The drawing under review shows one solid part. Ordinate dimensions are in mm from its lowest x, y, z. A direction names the side the tool comes from. Coordinates: 2 decimals unless noted, no trailing zeros. Order: outer loops, then holes, each group sorted by start corner. A loop starts at its lowest first (then second) coordinate and runs counter-clockwise, first axis right, second up. Notation, with made-up numbers: (37, 62.5) -> (61, 62.5) arc R12 cw to (61, 66.5) -> close; hole circle Ø11 at (21, 15.25). An arc over 180 degrees is marked (long way). Use a Markdown table: item, result. Add a question column.
Q1. Add section D-D (x = 21). State the section outline as (y, z) points (3 decimals), then the cut area to 3 significant figures.
Q2. Wall thickness on probe 1 along Y at (x, z) = (13, 9.25) (3 decimals); probe 2 along Z at (x, y) = (4, 6); probe 3 along Z at (x, y) = (19, 57): over which ranges is each line inside the solid? List them lowest first.
Q3. Insertion check: pin 1 (5 mm diameter, centred on y = 41, z = 8, fed in from -X); pin 2 (6 mm diameter, centred on y = 27, z = 8.5, fed in from +X); pin 3 (8 mm diameter, centred on y = 61.5, z = 6, fed in from -X); pin 4 (1 mm diameter, centred on x = 11.5, y = 42.5, fed in from +Z). Each pin has a flat end and moves straight along its axis. Give the tip position at first contact, or say it passes through.
Q4. Add section C-C (y = 10). State the section outline as (x, z) points.
Q5. Machinability: for the marked faces 3, 4 and 5, which of the approach directions +Z, -Z, +X, -X, +Y, -Y give a long, thin tool a straight path to every point of the face, cutting with its end or side? Answer none if there is none.
Q6. The part is to be moulded in two halves that separate along Y. For the marked faces 1 and 2, say which applies: pulls with the +Y half, pulls with the -Y half, needs draft (parallel to the pull), parting line crosses it, or undercut.
Q7. Add section A-A (z = 5). Count the separate pieces of the cut face and the enclosed holes in it, then the cut area to 3 significant figures.
Q8. Add section B-B (x = 13). State the section outline as (y, z) points (3 decimals).
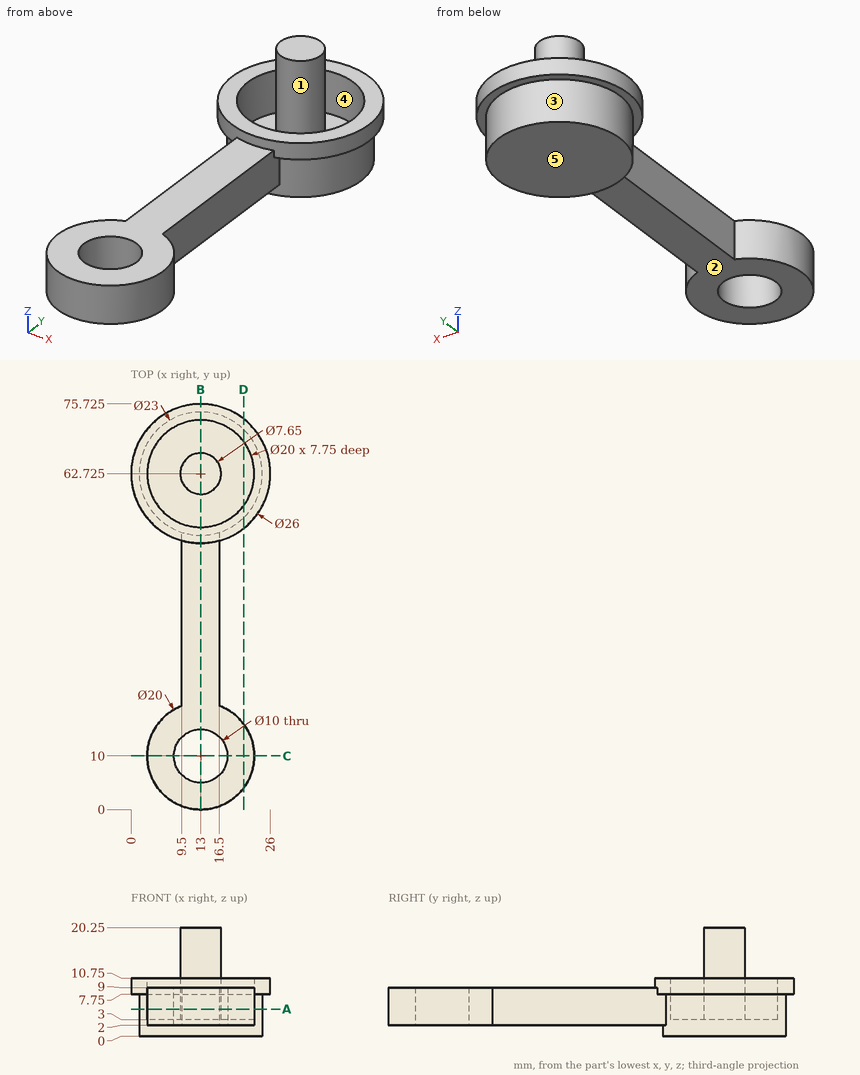
Established:
| question | item | result |
|---|---|---|
| 1 | outline | (4, 2) -> (16, 2) -> (16, 9) -> (4, 9) -> close; (52.478, 7.75) -> (54.464, 7.75) -> (54.464, 0) -> (70.986, 0) -> (70.986, 7.75) -> (72.972, 7.75) -> (72.972, 10.75) -> (68.725, 10.75) -> (68.725, 3) -> (56.725, 3) -> (56.725, 10.75) -> (52.478, 10.75) -> close |
| 1 | area | 181 mm^2 |
| 2 | probe 1 | 49.725 to 52.725, 58.9 to 66.55, 72.725 to 75.725 |
| 2 | probe 2 | 2 to 9 |
| 2 | probe 3 | 0 to 3 |
| 3 | pin 1 | x = 9.5 |
| 3 | pin 2 | x = 16.5 |
| 3 | pin 3 | x = 0 |
| 3 | pin 4 | z = 9 |
| 4 | outline | (3, 2) -> (8, 2) -> (8, 9) -> (3, 9) -> close; (18, 2) -> (23, 2) -> (23, 9) -> (18, 9) -> close |
| 5 | face 3 | -Z |
| 5 | face 4 | +Z |
| 5 | face 5 | -Z, +X, -X, +Y, -Y |
| 6 | face 1 | undercut |
| 6 | face 2 | needs draft |
| 7 | separate pieces | 2 |
| 7 | enclosed holes | 2 |
| 7 | area | 604 mm^2 |
| 8 | outline | (0, 2) -> (5, 2) -> (5, 9) -> (0, 9) -> close; (15, 2) -> (51.225, 2) -> (51.225, 0) -> (74.225, 0) -> (74.225, 7.75) -> (75.725, 7.75) -> (75.725, 10.75) -> (72.725, 10.75) -> (72.725, 3) -> (66.55, 3) -> (66.55, 20.25) -> (58.9, 20.25) -> (58.9, 3) -> (52.725, 3) -> (52.725, 10.75) -> (49.725, 10.75) -> (49.725, 9) -> (15, 9) -> close |
